Here's how the part is built. I have some questions about the finished solid (model axes, mm). Round coordinates to 2 decimals unless told otherwise and drop trailing zeros. Write each loop counter-clockwise with the first axis right and the second up, starting at its lowest first coordinate (ties: lowest second). Pieces come first, ordered by that corner, then holes. Notation, with made-up numbers: (-19, -19) -> (15, -19) arc R37 cw to (15, 18) -> close; hole circle Ø3 at (82.25, -24). An arc over 180 degrees is marked (long way). Put each result on its own line as item: value. Start each with the question number.
1) I want a section at A-A, the plane x = 0. List the corners of the cut face in (y, z) for me.
2) If I drill on line 1 along X through (y, z) = (0, 1169); line 2 along X through (y, z) = (7, 1173), over which ranges is the centre line in solid material (lowest first)? Write a range as [from, to].
3) Will these pins go through, and if not, where does the flat tip stop? P1, Ø3, axis at x = 0, y = 0, coming from the +Z side (3 decimals); P2, Ø2, axis at y = 2.5, z = 1200.5, coming from the -X side; P3, Ø0.6, axis at x = -9, z = 1151.5, coming from the -Y side; P4, Ø5, axis at y = -0.5, z = 1188, coming from the +X side.
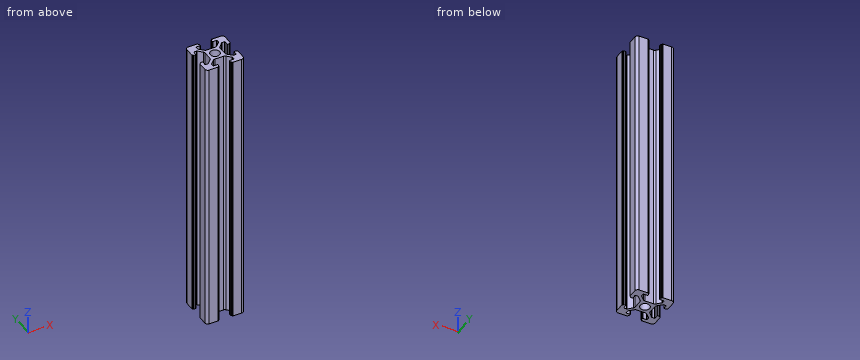
from build123d import *

# Parameters (mm, degrees)
SKETCH_1_R         = 2.5
EXTRUDE_1_DEPTH    = 1220
SKETCH1_R          = 16.771487081
CUT_EXTRUDE1_DEPTH = 1075


with BuildPart() as part:
    # 草图1 → 凸台-拉伸1 (new body)
    with BuildSketch(Plane.XY):
        with BuildLine():
            Line((-8.502261885, -10.002261885), (-3.85, -10.002261885))
            ThreePointArc((-3.85, -10.002261885), (-3.673223305, -9.929038581), (-3.6, -9.752261885))
            Line((-3.6, -9.752261885), (-3.6, -9.502261885))
            Line((-3.6, -9.502261885), (-3.35, -9.502261885))
            ThreePointArc((-3.35, -9.502261885), (-3.173223305, -9.429038581), (-3.1, -9.252261885))
            Line((-3.1, -9.252261885), (-3.1, -8.45))
            ThreePointArc((-3.1, -8.45), (-3.173223305, -8.273223305), (-3.35, -8.2))
            Line((-3.35, -8.2), (-5.25, -8.2))
            ThreePointArc((-5.25, -8.2), (-5.426776695, -8.126776695), (-5.5, -7.95))
            Line((-5.5, -7.95), (-5.5, -6.664213562))
            ThreePointArc((-5.5, -6.664213562), (-5.480969883, -6.568542704), (-5.426776695, -6.487436867))
            Line((-5.426776695, -6.487436867), (-3.278679656, -4.339339828))
            ThreePointArc((-3.278679656, -4.339339828), (-2.792044633, -4.014180701), (-2.218019485, -3.9))
            Line((-2.218019485, -3.9), (2.218019485, -3.9))
            ThreePointArc((2.218019485, -3.9), (2.792044633, -4.014180701), (3.278679656, -4.339339828))
            Line((3.278679656, -4.339339828), (5.426776695, -6.487436867))
            ThreePointArc((5.426776695, -6.487436867), (5.480969883, -6.568542704), (5.5, -6.664213562))
            Line((5.5, -6.664213562), (5.5, -7.95))
            ThreePointArc((5.5, -7.95), (5.426776695, -8.126776695), (5.25, -8.2))
            Line((5.25, -8.2), (3.35, -8.2))
            ThreePointArc((3.35, -8.2), (3.173223305, -8.273223305), (3.1, -8.45))
            Line((3.1, -8.45), (3.1, -9.252261885))
            ThreePointArc((3.1, -9.252261885), (3.173223305, -9.429038581), (3.35, -9.502261885))
            Line((3.35, -9.502261885), (3.6, -9.502261885))
            Line((3.6, -9.502261885), (3.6, -9.752261885))
            ThreePointArc((3.6, -9.752261885), (3.673223305, -9.929038581), (3.85, -10.002261885))
            Line((3.85, -10.002261885), (8.502261885, -10.002261885))
            ThreePointArc((8.502261885, -10.002261885), (9.562922057, -9.562922057), (10.002261885, -8.502261885))
            Line((10.002261885, -8.502261885), (10.002261885, -3.85))
            ThreePointArc((10.002261885, -3.85), (9.929038581, -3.673223305), (9.752261885, -3.6))
            Line((9.752261885, -3.6), (9.502261885, -3.6))
            Line((9.502261885, -3.6), (9.502261885, -3.35))
            ThreePointArc((9.502261885, -3.35), (9.429038581, -3.173223305), (9.252261885, -3.1))
            Line((9.252261885, -3.1), (8.45, -3.1))
            ThreePointArc((8.45, -3.1), (8.273223305, -3.173223305), (8.2, -3.35))
            Line((8.2, -3.35), (8.2, -5.25))
            ThreePointArc((8.2, -5.25), (8.126776695, -5.426776695), (7.95, -5.5))
            Line((7.95, -5.5), (6.664213562, -5.5))
            ThreePointArc((6.664213562, -5.5), (6.568542704, -5.480969883), (6.487436867, -5.426776695))
            Line((6.487436867, -5.426776695), (4.339339828, -3.278679656))
            ThreePointArc((4.339339828, -3.278679656), (4.014180701, -2.792044633), (3.9, -2.218019485))
            Line((3.9, -2.218019485), (3.9, 2.218019485))
            ThreePointArc((3.9, 2.218019485), (4.014180701, 2.792044633), (4.339339828, 3.278679656))
            Line((4.339339828, 3.278679656), (6.487436867, 5.426776695))
            ThreePointArc((6.487436867, 5.426776695), (6.568542704, 5.480969883), (6.664213562, 5.5))
            Line((6.664213562, 5.5), (7.95, 5.5))
            ThreePointArc((7.95, 5.5), (8.126776695, 5.426776695), (8.2, 5.25))
            Line((8.2, 5.25), (8.2, 3.35))
            ThreePointArc((8.2, 3.35), (8.273223305, 3.173223305), (8.45, 3.1))
            Line((8.45, 3.1), (9.252261885, 3.1))
            ThreePointArc((9.252261885, 3.1), (9.429038581, 3.173223305), (9.502261885, 3.35))
            Line((9.502261885, 3.35), (9.502261885, 3.6))
            Line((9.502261885, 3.6), (9.752261885, 3.6))
            ThreePointArc((9.752261885, 3.6), (9.929038581, 3.673223305), (10.002261885, 3.85))
            Line((10.002261885, 3.85), (10.002261885, 8.502261885))
            ThreePointArc((10.002261885, 8.502261885), (9.562922057, 9.562922057), (8.502261885, 10.002261885))
            Line((8.502261885, 10.002261885), (3.85, 10.002261885))
            ThreePointArc((3.85, 10.002261885), (3.673223305, 9.929038581), (3.6, 9.752261885))
            Line((3.6, 9.752261885), (3.6, 9.502261885))
            Line((3.6, 9.502261885), (3.35, 9.502261885))
            ThreePointArc((3.35, 9.502261885), (3.173223305, 9.429038581), (3.1, 9.252261885))
            Line((3.1, 9.252261885), (3.1, 8.45))
            ThreePointArc((3.1, 8.45), (3.173223305, 8.273223305), (3.35, 8.2))
            Line((3.35, 8.2), (5.25, 8.2))
            ThreePointArc((5.25, 8.2), (5.426776695, 8.126776695), (5.5, 7.95))
            Line((5.5, 7.95), (5.5, 6.664213562))
            ThreePointArc((5.5, 6.664213562), (5.480969883, 6.568542704), (5.426776695, 6.487436867))
            Line((5.426776695, 6.487436867), (3.278679656, 4.339339828))
            ThreePointArc((3.278679656, 4.339339828), (2.792044633, 4.014180701), (2.218019485, 3.9))
            Line((2.218019485, 3.9), (-2.218019485, 3.9))
            ThreePointArc((-2.218019485, 3.9), (-2.792044633, 4.014180701), (-3.278679656, 4.339339828))
            Line((-3.278679656, 4.339339828), (-5.426776695, 6.487436867))
            ThreePointArc((-5.426776695, 6.487436867), (-5.480969883, 6.568542704), (-5.5, 6.664213562))
            Line((-5.5, 6.664213562), (-5.5, 7.95))
            ThreePointArc((-5.5, 7.95), (-5.426776695, 8.126776695), (-5.25, 8.2))
            Line((-5.25, 8.2), (-3.35, 8.2))
            ThreePointArc((-3.35, 8.2), (-3.173223305, 8.273223305), (-3.1, 8.45))
            Line((-3.1, 8.45), (-3.1, 9.252261885))
            ThreePointArc((-3.1, 9.252261885), (-3.173223305, 9.429038581), (-3.35, 9.502261885))
            Line((-3.35, 9.502261885), (-3.6, 9.502261885))
            Line((-3.6, 9.502261885), (-3.6, 9.752261885))
            ThreePointArc((-3.6, 9.752261885), (-3.673223305, 9.929038581), (-3.85, 10.002261885))
            Line((-3.85, 10.002261885), (-8.502261885, 10.002261885))
            ThreePointArc((-8.502261885, 10.002261885), (-9.562922057, 9.562922057), (-10.002261885, 8.502261885))
            Line((-10.002261885, 8.502261885), (-10.002261885, 3.85))
            ThreePointArc((-10.002261885, 3.85), (-9.929038581, 3.673223305), (-9.752261885, 3.6))
            Line((-9.752261885, 3.6), (-9.502261885, 3.6))
            Line((-9.502261885, 3.6), (-9.502261885, 3.35))
            ThreePointArc((-9.502261885, 3.35), (-9.429038581, 3.173223305), (-9.252261885, 3.1))
            Line((-9.252261885, 3.1), (-8.45, 3.1))
            ThreePointArc((-8.45, 3.1), (-8.273223305, 3.173223305), (-8.2, 3.35))
            Line((-8.2, 3.35), (-8.2, 5.25))
            ThreePointArc((-8.2, 5.25), (-8.126776695, 5.426776695), (-7.95, 5.5))
            Line((-7.95, 5.5), (-6.664213562, 5.5))
            ThreePointArc((-6.664213562, 5.5), (-6.568542704, 5.480969883), (-6.487436867, 5.426776695))
            Line((-6.487436867, 5.426776695), (-4.339339828, 3.278679656))
            ThreePointArc((-4.339339828, 3.278679656), (-4.014180701, 2.792044633), (-3.9, 2.218019485))
            Line((-3.9, 2.218019485), (-3.9, -2.218019485))
            ThreePointArc((-3.9, -2.218019485), (-4.014180701, -2.792044633), (-4.339339828, -3.278679656))
            Line((-4.339339828, -3.278679656), (-6.487436867, -5.426776695))
            ThreePointArc((-6.487436867, -5.426776695), (-6.568542704, -5.480969883), (-6.664213562, -5.5))
            Line((-6.664213562, -5.5), (-7.95, -5.5))
            ThreePointArc((-7.95, -5.5), (-8.126776695, -5.426776695), (-8.2, -5.25))
            Line((-8.2, -5.25), (-8.2, -3.35))
            ThreePointArc((-8.2, -3.35), (-8.273223305, -3.173223305), (-8.45, -3.1))
            Line((-8.45, -3.1), (-9.252261885, -3.1))
            ThreePointArc((-9.252261885, -3.1), (-9.429038581, -3.173223305), (-9.502261885, -3.35))
            Line((-9.502261885, -3.35), (-9.502261885, -3.6))
            Line((-9.502261885, -3.6), (-9.752261885, -3.6))
            ThreePointArc((-9.752261885, -3.6), (-9.929038581, -3.673223305), (-10.002261885, -3.85))
            Line((-10.002261885, -3.85), (-10.002261885, -8.502261885))
            ThreePointArc((-10.002261885, -8.502261885), (-9.562922057, -9.562922057), (-8.502261885, -10.002261885))
        make_face()
        Circle(SKETCH_1_R, mode=Mode.SUBTRACT)
    extrude(amount=EXTRUDE_1_DEPTH)

    # Sketch1 → Cut-Extrude1 (cut, through all)
    with BuildSketch(Plane.XY.offset(1074)):
        Circle(SKETCH1_R)
    extrude(amount=-CUT_EXTRUDE1_DEPTH, mode=Mode.SUBTRACT)


solid = part.part
Findings:
1. outline: (-3.9, 1074) -> (-2.5, 1074) -> (-2.5, 1220) -> (-3.9, 1220) -> close; (2.5, 1074) -> (3.9, 1074) -> (3.9, 1220) -> (2.5, 1220) -> close
2. line 1: x = [-3.9, -2.5], [2.5, 3.9]
2. line 2: x = [-10, -5.5], [5.5, 10]
3. P1: passes through
3. P2: stops at x = -9.5
3. P3: stops at y = -9.99
3. P4: stops at x = 4.12
